For this review, use the dimensioned drawing (mm, ordinates from the lowest corner) and the shaded views. A direction names the side the tool comes from. Coordinates: 2 decimals unless noted, no trailing zeros. Loops run counter-clockwise (first coordinate to the right, second up) from the corner with the lowest first, then second, coordinate; pieces in that order, holes last. Notation, with made-up numbers: (37, 74) -> (56, 74) arc R20 cw to (56, 98) -> close; hole circle Ø8 at (30.25, 26). An arc over 180 degrees is marked (long way). Answer as a JSON object with one key per item and string values.
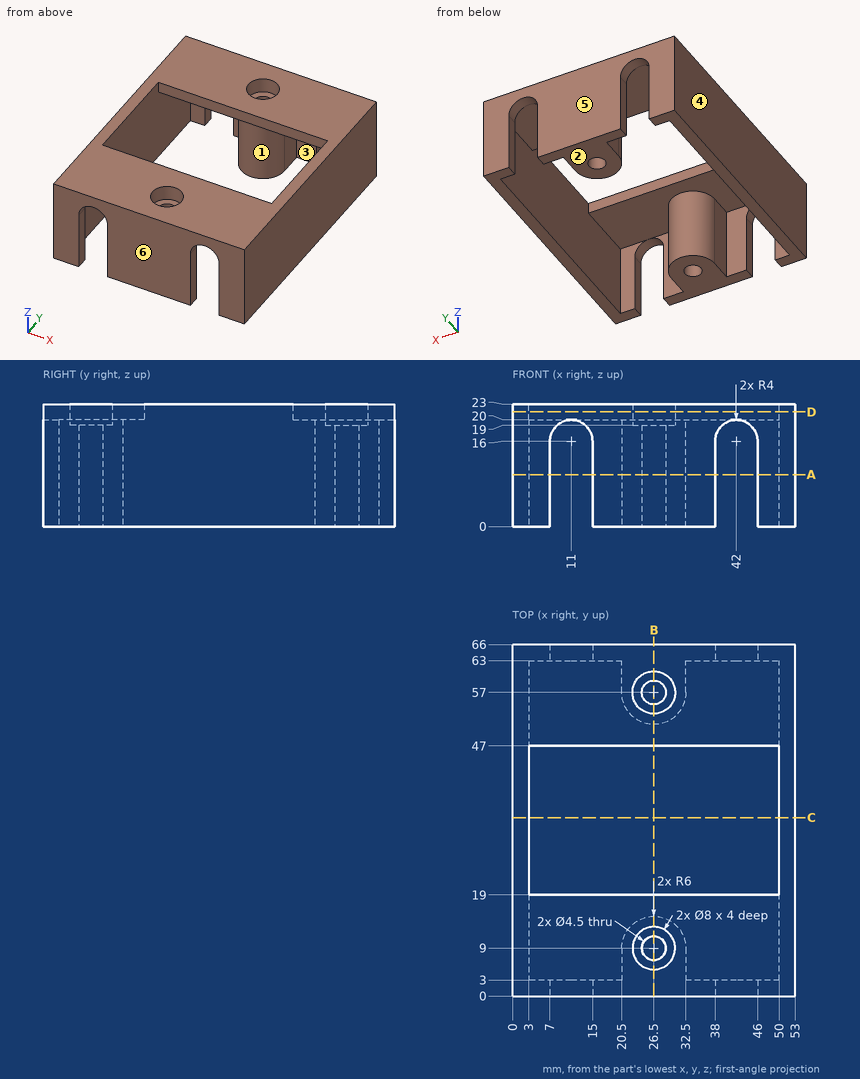
1) Clearance check with flat-ended pins moving along their axes: pin 1 Ø10 at (x, y) = (19.5, 45.5) entering from -Z; pin 2 Ø4 at (x, y) = (28, 9) entering from +Z. State where each tip first meets the part, or that it passes through.
Completed:
{"pin 1": "z = 20", "pin 2": "z = 19"}
2) Add section A-A, the plane z = 9.75. Count the separate pieces of the cut face and the enclosed holes in it, and give its area (3 significant figures).
Completed:
{"separate pieces": "4", "enclosed holes": "2", "area": "807 mm²"}
3) For the marked faces 1 and 2, list the 3-axis set-ups (+Z, -Z, +X, -X, +Y, -Y) from which the entire face can be reached by the end or side of a thin tool; tool diameter is ignored.
Completed:
{"face 1": "-Z", "face 2": "-Z, +X, -X, +Y, -Y"}
4) The part is to be moulded in two halves that separate along Y. For the marked faces 3, 4, 5 and 6, say which applies: pulls with the +Y half, pulls with the -Y half, needs draft (parallel to the pull), parting line crosses it, or undercut.
Completed:
{"face 3": "undercut", "face 4": "needs draft", "face 5": "pulls with the +Y half", "face 6": "pulls with the -Y half"}
5) Add section C-C, the plane y = 33.5. Give the boundary of the cut face in (x, z).
Completed:
{"outline": "(0, 0) -> (3, 0) -> (3, 23) -> (0, 23) -> close; (50, 0) -> (53, 0) -> (53, 23) -> (50, 23) -> close"}
6) Wall thickness on probe 1 along X at (y, z) = (41, 17); probe 2 along Y at (x, z) = (26.5, 12); probe 3 along X at (y, z) = (9, 20.6): over which ranges is each line inside the solid? List them lowest first.
Completed:
{"probe 1": "0 to 3, 50 to 53", "probe 2": "0 to 6.75, 11.25 to 15, 51 to 54.75, 59.25 to 66", "probe 3": "0 to 22.5, 30.5 to 53"}
7) Add section D-D, the plane z = 21.5. Give the boundary of the cut face in (x, y).
Completed:
{"outline": "(0, 0) -> (53, 0) -> (53, 66) -> (0, 66) -> close; hole (3, 19) -> (50, 19) -> (50, 47) -> (3, 47) -> close; hole circle Ø8 at (26.5, 9); hole circle Ø8 at (26.5, 57)"}
8) Add section B-B, the plane x = 26.5. Give the boundary of the cut face in (y, z).
Completed:
{"outline": "(0, 0) -> (6.75, 0) -> (6.75, 19) -> (5, 19) -> (5, 23) -> (0, 23) -> close; (11.25, 0) -> (15, 0) -> (15, 20) -> (19, 20) -> (19, 23) -> (13, 23) -> (13, 19) -> (11.25, 19) -> close; (47, 20) -> (51, 20) -> (51, 0) -> (54.75, 0) -> (54.75, 19) -> (53, 19) -> (53, 23) -> (47, 23) -> close; (59.25, 0) -> (66, 0) -> (66, 23) -> (61, 23) -> (61, 19) -> (59.25, 19) -> close"}
